Source: three-view drawing plus pictorial views. Frame: mm from the lowest corner of the part. A direction names the side the tool comes from. Coordinates: 2 decimals unless noted, no trailing zeros. Write each loop counter-clockwise with the first axis right and the second up, starting at its lowest first coordinate (ties: lowest second). Pieces come first, ordered by that corner, then holes. Notation, with made-up numbers: (7, -32) - (54, -32) arc R19 ccw to (54, -7) - close; hole circle Ø3 at (18, -21). An arc over 180 degrees is marked (long way). Put each result on its own line as item: value.
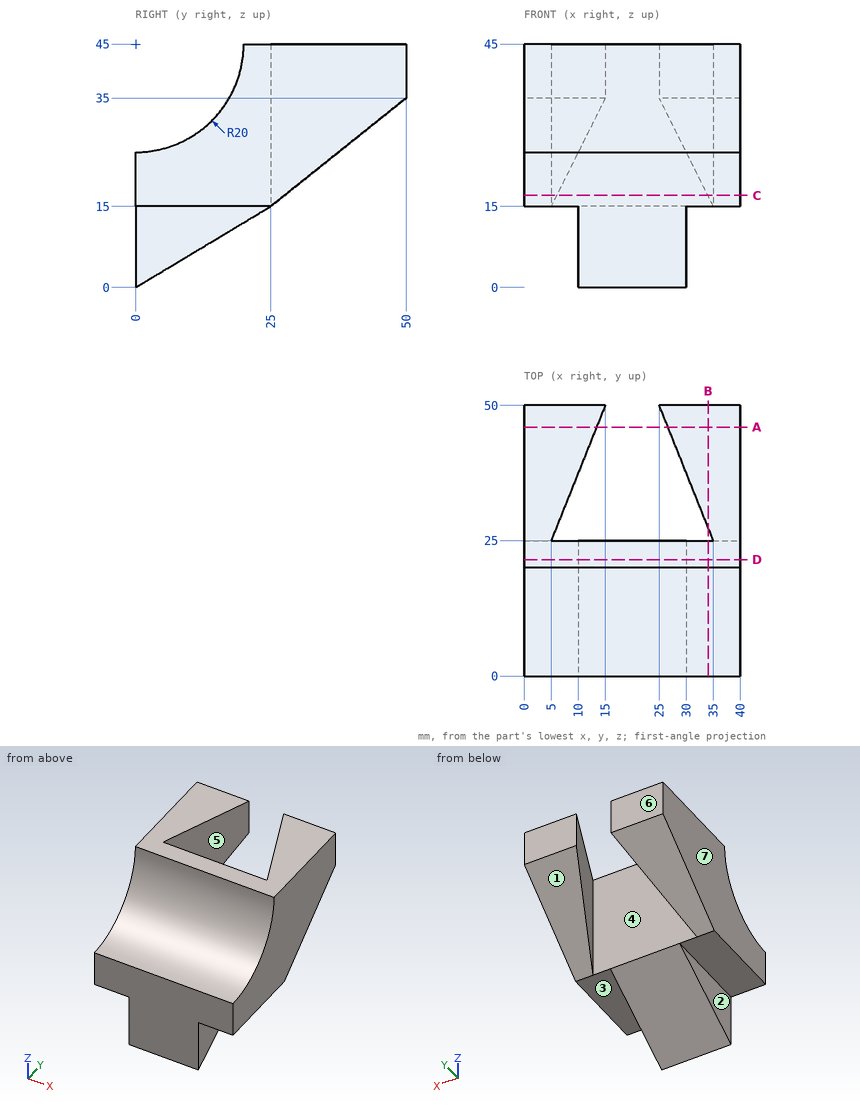
1. Section query B-B (x = 34). Return loops of the section in (y, z), then the cut area to 3 significant figures.
Answer below:
outline: (0, 15) - (25, 15) - (25, 45) - (20, 45) arc R20 cw to (0, 25) - close; (27.5, 17) - (50, 35) - (50, 45) - (27.5, 45) - close
area: 863 mm²
2. Ray query, probe 1 along Y at (x, z) = (16.5, 6); probe 2 along X at (y, z) = (33.5, 35); probe 3 along X at (y, z) = (5.5, 11.5). Return the intervals inside material, ascending. Write a range as from..to.
Answer below:
probe 1: y = 0..10
probe 2: x = 0..8.4, 31.6..40
probe 3: x = 10..30
3. Section query D-D (y = 21.5). Return loops of the section in (x, z).
Answer below:
outline: (0, 15) - (10, 15) - (10, 12.9) - (30, 12.9) - (30, 15) - (40, 15) - (40, 45) - (0, 45) - close
4. Section query C-C (z = 17). Return loops of the section in (x, y), then the cut area to 3 significant figures.
Answer below:
outline: (0, 0) - (40, 0) - (40, 27.5) - (34, 27.5) - (35, 25) - (5, 25) - (6, 27.5) - (0, 27.5) - close
area: 1,030 mm²
5. Section query A-A (y = 46). Return loops of the section in (x, z), then the cut area to 3 significant figures.
Answer below:
outline: (0, 31.8) - (13.4, 31.8) - (13.4, 45) - (0, 45) - close; (26.6, 31.8) - (40, 31.8) - (40, 45) - (26.6, 45) - close
area: 354 mm²
6. Set-up query: the marked faces 1, 2 and 3. Return all of +Z, -Z, +X, -X, +Y, -Y with unobstructed straight access to the full face (end or side cutting, diameter ignored); none if empty.
Answer below:
face 1: -Z, +X, -X, +Y
face 2: -Z, -X, +Y, -Y
face 3: -Z, +X, +Y, -Y
7. Mould query, pull axis X, two halves, no side actions, for the marked faces 4, 5, 6 and 7. Classes: +X half, -X half, draft (parallel to the pull), parting line (faces both ways), or undercut.
Answer below:
face 4: undercut
face 5: undercut
face 6: draft
face 7: -X half
8. Pin query (flat end, axial travel): pin 1 Ø4 at (x, y) = (19.5, 6.5) entering from -Z; pin 2 Ø1 at (x, y) = (16, 24) entering from -Z; pin 3 Ø10 at (x, z) = (33.5, 15.5) entering from +Y (3 decimals). Return the tip coordinate at first contact, or that it passes through.
Answer below:
pin 1: stops at z = 2.7
pin 2: stops at z = 14.1
pin 3: stops at y = 31.875
